```python
from build123d import *

# Parameters (mm, degrees)
F0_W     = 22.6
F0_H     = 12
F1_DEPTH = 22.5
F2_R     = 6
F3_DEPTH = 4.3
F4_R     = 2.3
F5_DEPTH = 2
F6_R     = 2.5
F7_DEPTH = 5


with BuildPart() as f1:
    # F0 (on Top) → F1 (new body)
    with BuildSketch(Plane.XY):
        Rectangle(F0_W, F0_H)
    extrude(amount=F1_DEPTH)

    # F2 (on face) → F3 (join)
    with BuildSketch(Plane.XY.offset(22.5)):
        with Locations((-5.3, 0)):
            Circle(F2_R)
    extrude(amount=F3_DEPTH)

    # F4 (on face) → F5 (join)
    with BuildSketch(Plane.XY.offset(26.8)):
        with Locations((-5.3, 0)):
            Circle(F4_R)
    extrude(amount=F5_DEPTH)

    # F6 (on face) → F7 (join)
    with BuildSketch(Plane.XY.offset(26.8)):
        with Locations((0.7, 0)):
            Circle(F6_R)
    extrude(amount=-F7_DEPTH)


solid = f1.part
```
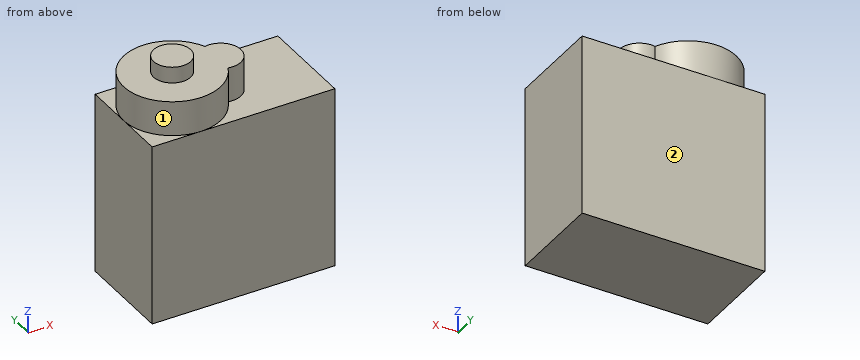
Verification items for the finished model (mm, model axes). Face numbers are marked on the shaded views. A direction names the side the tool comes from. Coordinates: 2 decimals unless noted, no trailing zeros. Loops run counter-clockwise (first coordinate to the right, second up) from the corner with the lowest first, then second, coordinate; pieces in that order, holes last. Notation, with made-up numbers: (29.5, -35) -> (35.5, -35) arc R23 cw to (35.5, 3) -> close; hole circle Ø3 at (67, 39). An arc over 180 degrees is marked (long way). Answer in a Markdown table with one row per item. Add a question column.
1. Section check B-B, the plane y = 1.25. Enter the section's corners in (x, z), then the cut area to 3 significant figures.
2. Depth check by flat-ended pin: P1, Ø3, axis at x = -9.5, y = 4.5, coming from the +Z side. Enter the tip coordinate at first touch or a pass-through.
3. Section check D-D, the plane y = -3. Enter the section's corners in (x, z).
4. Section check C-C, the plane x = -3.5. Enter the section's corners in (y, z), then the cut area to 3 significant figures.
5. Access from +Z, -Z, +X, -X, +Y, -Y to the whole of each face (thin tool, end or side, straight path). Record for the marked faces 1 and 2.
6. Section check A-A, the plane x = 0.7. Enter the section's corners in (y, z).
7. Material ranges on probe 1 along Z at (x, y) = (8, -3); probe 2 along Z at (x, y) = (-1, -2.5); probe 3 along X at (y, z) = (0.5, 23.75), recorded low to high. Write a range as [from, to].
Derived:
| question | item | result |
|---|---|---|
| 1 | outline | (-11.3, 0) -> (11.3, 0) -> (11.3, 22.5) -> (2.87, 22.5) -> (2.87, 26.8) -> (-3.37, 26.8) -> (-3.37, 28.8) -> (-7.23, 28.8) -> (-7.23, 26.8) -> (-11.17, 26.8) -> (-11.17, 22.5) -> (-11.3, 22.5) -> close |
| 1 | area | 577 mm² |
| 2 | P1 | stops at z = 26.8 |
| 3 | outline | (-11.3, 0) -> (11.3, 0) -> (11.3, 22.5) -> (-0.1, 22.5) -> (-0.1, 26.8) -> (-10.5, 26.8) -> (-10.5, 22.5) -> (-11.3, 22.5) -> close |
| 4 | outline | (-6, 0) -> (6, 0) -> (6, 22.5) -> (5.72, 22.5) -> (5.72, 26.8) -> (1.43, 26.8) -> (1.43, 28.8) -> (-1.43, 28.8) -> (-1.43, 26.8) -> (-5.72, 26.8) -> (-5.72, 22.5) -> (-6, 22.5) -> close |
| 4 | area | 325 mm² |
| 5 | face 1 | +Z |
| 5 | face 2 | +Z, -Z, +X, -X, +Y |
| 6 | outline | (-6, 0) -> (6, 0) -> (6, 22.5) -> (2.5, 22.5) -> (2.5, 26.8) -> (-2.5, 26.8) -> (-2.5, 22.5) -> (-6, 22.5) -> close |
| 7 | probe 1 | z = [0, 22.5] |
| 7 | probe 2 | z = [0, 26.8] |
| 7 | probe 3 | x = [-11.28, 3.15] |
